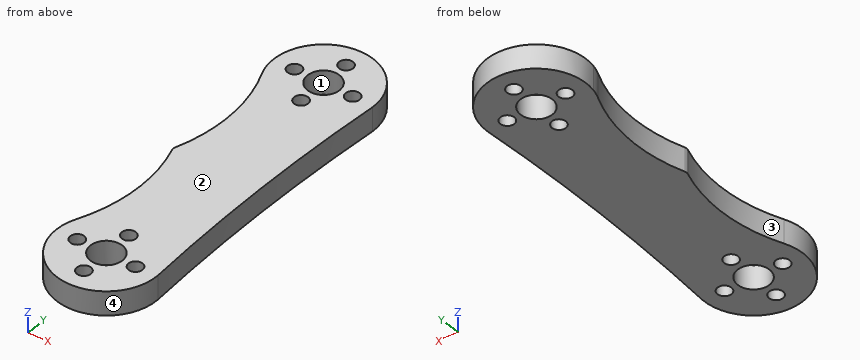
```python
from build123d import *

# Parameters (mm, degrees)
SKETCH1_W           = 30
SKETCH1_H           = 100
BOSS_EXTRUDE1_DEPTH = 6
SKETCH2_W           = 30
SKETCH2_H           = 100
SKETCH2_R           = 4
SKETCH2_R_2         = 1.75
CUT_EXTRUDE1_DEPTH  = 6


with BuildPart() as part:
    # Sketch1 → Boss-Extrude1 (new body)
    with BuildSketch(Plane.XY):
        Rectangle(SKETCH1_W, SKETCH1_H)
    extrude(amount=BOSS_EXTRUDE1_DEPTH)

    # Sketch2 → Cut-Extrude1 (cut)
    # profile 1 of 11: a face of its own
    with BuildSketch(Plane(origin=(0, 0, 0), x_dir=(-1, 0, 0), z_dir=(0, 0, -1))):
        Rectangle(SKETCH2_W, SKETCH2_H)
        with BuildLine():
            ThreePointArc((-11.532456366, 35.433789865), (-10.931527192, 0.86004689), (-12.814966119, -33.667586637))
            ThreePointArc((-12.814966119, -33.667586637), (1.804726533, -46.658495876), (11.190763167, -29.50036508))
            ThreePointArc((11.190763167, -29.50036508), (8.075913228, -14.826459902), (10.585521288, -0.037016008))
            ThreePointArc((10.585521288, -0.037016008), (10.679689693, 0.458946393), (10.603989757, 0.958061522))
            ThreePointArc((10.603989757, 0.958061522), (8.644900126, 15.830443683), (12.302107664, 30.37866063))
            ThreePointArc((12.302107664, 30.37866063), (12.787952713, 31.585012611), (13.145828199, 32.835314836))
            ThreePointArc((13.145828199, 32.835314836), (2.274693549, 48.076541281), (-11.532456366, 35.433789865))
        make_face(mode=Mode.SUBTRACT)
    # profile 2 of 11: a face of its own
    with BuildSketch(Plane(origin=(0, 0, 0), x_dir=(-1, 0, 0), z_dir=(0, 0, -1))):
        with Locations((0.965754671, 35.645263027)):
            Circle(SKETCH2_R)
    # profile 3 of 11: a face of its own
    with BuildSketch(Plane(origin=(0, 0, 0), x_dir=(-1, 0, 0), z_dir=(0, 0, -1))):
        with Locations((1.100290264, 42.894014656)):
            Circle(SKETCH2_R_2)
    # profile 4 of 11: a face of its own
    with BuildSketch(Plane(origin=(0, 0, 0), x_dir=(-1, 0, 0), z_dir=(0, 0, -1))):
        with Locations((8.214506299, 35.510727434)):
            Circle(SKETCH2_R_2)
    # profile 5 of 11: a face of its own
    with BuildSketch(Plane(origin=(0, 0, 0), x_dir=(-1, 0, 0), z_dir=(0, 0, -1))):
        with Locations((0.831219078, 28.396511399)):
            Circle(SKETCH2_R_2)
    # profile 6 of 11: a face of its own
    with BuildSketch(Plane(origin=(0, 0, 0), x_dir=(-1, 0, 0), z_dir=(0, 0, -1))):
        with Locations((-6.282996958, 35.77979862)):
            Circle(SKETCH2_R_2)
    # profile 7 of 11: a face of its own
    with BuildSketch(Plane(origin=(0, 0, 0), x_dir=(-1, 0, 0), z_dir=(0, 0, -1))):
        with Locations((-0.333209676, -34.342683732)):
            Circle(SKETCH2_R)
    # profile 8 of 11: a face of its own
    with BuildSketch(Plane(origin=(0, 0, 0), x_dir=(-1, 0, 0), z_dir=(0, 0, -1))):
        with Locations((-0.198674083, -27.093932103)):
            Circle(SKETCH2_R_2)
    # profile 9 of 11: a face of its own
    with BuildSketch(Plane(origin=(0, 0, 0), x_dir=(-1, 0, 0), z_dir=(0, 0, -1))):
        with Locations((6.915541953, -34.477219325)):
            Circle(SKETCH2_R_2)
    # profile 10 of 11: a face of its own
    with BuildSketch(Plane(origin=(0, 0, 0), x_dir=(-1, 0, 0), z_dir=(0, 0, -1))):
        with Locations((-7.581961304, -34.208148139)):
            Circle(SKETCH2_R_2)
    # profile 11 of 11: a face of its own
    with BuildSketch(Plane(origin=(0, 0, 0), x_dir=(-1, 0, 0), z_dir=(0, 0, -1))):
        with Locations((-0.467745269, -41.591435361)):
            Circle(SKETCH2_R_2)
    extrude(amount=-CUT_EXTRUDE1_DEPTH, mode=Mode.SUBTRACT)


solid = part.part
```
Can you work these out from the model? Positions are in its coordinate system, mm. Face numbers are marked on the shaded views. Round coordinates to 2 decimals unless told otherwise and drop trailing zeros. Loops run counter-clockwise (first coordinate to the right, second up) from the corner with the lowest first, then second, coordinate; pieces in that order, holes last. Notation, with made-up numbers: (-29.75, 30) -> (11.25, 30) arc R27 cw to (11.25, 63) -> close; hole circle Ø8 at (30, -4). An arc over 180 degrees is marked (long way). One line per item, written item: value. Start each with the question number.
1. If we section it at C-C, the plane y = 19.5: Write out the boundary of the cut face in (x, z), then the cut area to 3 significant figures.
2. If we section it at B-B, the plane y = -19: Write out the boundary of the cut face in (x, z).
3. If we section it at A-A, the plane z = 4.5: Give the number of separate pieces and of enclosed holes in the cut face, then the cut area to 3 significant figures.
4. If I drill on probe 1 along Y at (x, z) = (2.25, 0.8); probe 2 along X at (y, z) = (-35.5, 2.5); probe 3 along X at (y, z) = (36.5, 2.85), over which ranges is the centre line in solid material (lowest first)?
5. If we mould it in two halves opening along X, with no side actions, what happens to the marked faces 1, 2, 3 and 4? For each: pulls with the +X half, pulls with the -X half, needs draft (parallel to the pull), parting line crosses it, or undercut.
6. For pin 1 (13 mm diameter, centred on x = -0.97, y = 35.65, fed in from -Z); pin 2 (3 mm diameter, centred on x = -0.83, y = 28.4, fed in from +Z); pin 3 (2 mm diameter, centred on y = 8, z = 4, fed in from +X), each with a flat end and sliding along its axis, tell me the tip position at first contact or that it passes through.
Calculated:
1. outline: (-9.03, 0) -> (10.95, 0) -> (10.95, 6) -> (-9.03, 6) -> close
1. area: 120 mm²
2. outline: (-8.38, 0) -> (11.71, 0) -> (11.71, 6) -> (-8.38, 6) -> close
3. separate pieces: 1
3. enclosed holes: 10
3. area: 1,790 mm²
4. probe 1: y = -46.69 to -37.85, -30.83 to 33.27, 38.02 to 47.72
4. probe 2: x = -12.11 to -8.34, -5.5 to -3.5, 4.16 to 6.4, 8.76 to 12.78
4. probe 3: x = -13.44 to -9.66, -6.77 to -4.87, 2.94 to 4.69, 7.88 to 11.5
5. face 1: undercut
5. face 2: needs draft
5. face 3: pulls with the -X half
5. face 4: parting line crosses it
6. pin 1: stops at z = 0
6. pin 2: passes through
6. pin 3: stops at x = 10.86
